from build123d import *

# Parameters (mm, degrees)
SKETCH1_W           = 55.5
SKETCH1_H           = 73.2
BOSS_EXTRUDE1_DEPTH = 4
SKETCH2_W           = 52.220028237
SKETCH2_H           = 5.163547568
BOSS_EXTRUDE2_DEPTH = 5
SKETCH3_W           = 43
SKETCH3_H           = 61
BOSS_EXTRUDE3_DEPTH = 3
SKETCH4_W           = 55.5
SKETCH4_H           = 73.2
BOSS_EXTRUDE4_DEPTH = 60


with BuildPart() as part:
    # Sketch1 → Boss-Extrude1 (new body)
    with BuildSketch(Plane.XY):
        Rectangle(SKETCH1_W, SKETCH1_H)
    extrude(amount=BOSS_EXTRUDE1_DEPTH)

    # Sketch2 → Boss-Extrude2 (add)
    with BuildSketch(Plane(origin=(0, 0, 0), x_dir=(-1, 0, 0), z_dir=(0, 0, -1))):
        with Locations((0.292276277, 32.734943074)):
            Rectangle(SKETCH2_W, SKETCH2_H)
    extrude(amount=BOSS_EXTRUDE2_DEPTH)

    # Sketch3 → Boss-Extrude3 (add)
    with BuildSketch(Plane.XY.offset(4)):
        Rectangle(SKETCH3_W, SKETCH3_H)
    extrude(amount=BOSS_EXTRUDE3_DEPTH)

    # Sketch4 → Boss-Extrude4 (add)
    with BuildSketch(Plane(origin=(0, 0, -5), x_dir=(-1, 0, 0), z_dir=(0, 0, -1))):
        Rectangle(SKETCH4_W, SKETCH4_H)
    extrude(amount=BOSS_EXTRUDE4_DEPTH)


solid = part.part
Work out the finished part from the listing and answer in its coordinate system (mm). A direction names the side the tool comes from. Give positions to 0.01 mm unless a question says otherwise; leave off trailing zeros. Order: outer loops, then holes, each group sorted by start corner. A loop starts at its lowest first (then second) coordinate and runs counter-clockwise, first axis right, second up. Notation, with made-up numbers: (-32, -29) - (-28, -29) arc R17 ccw to (-28, 2) - close; hole circle Ø3 at (33.25, 37). An arc over 180 degrees is marked (long way). Answer as CSV lines item,"result". Start each with the question number.
Q1. Find the intervals of material crossed by L1, parallel to Z at x = -7.5, y = 20; L2, parallel to Z at x = -25, y = -19; L3, parallel to Z at x = 14, y = 34.5, in increasing order. Write a range as [from, to].
Q2. The part is cut by section A-A (y = 14). Write down the section's boundary in (x, z), then the cut area to 3 significant figures.
Q3. The part is cut by section B-B (x = 24). Write down the section's boundary in (y, z), then the cut area to 3 significant figures.
Q4. Given pin 1 Ø5.5 at (y, z) = (33.5, -2) entering from -X; pin 2 Ø2.5 at (x, z) = (9.5, -2) entering from +Y; pin 3 Ø2.5 at (x, z) = (-8.5, 6) entering from -Y; pin 4 Ø3.5 at (y, z) = (2, 6) entering from -X, each flat-ended and moving along its own axis, determine where each tip first touches the part or whether it passes through.
Q5. The part is cut by section D-D (x = -5). Write down the section's boundary in (y, z), then the cut area to 3 significant figures.
Q6. For faces 1 (the face through (-21.5, 0, 5)), 2 (the face through (0, 35.317, -2)), 3 (the face through (0, 30.5, 5)), 4 (the face through (25.818, 33, -2)), 5 (the face through (21.5, 0, 5)), determine the directions among +Z, -Z, +X, -X, +Y, -Y from which every point of the face is accessible in a straight line to the end or side of a thin tool.
Q7. The mould has two halves that part along Z. Classify faces 6 (the face through (0, 1, -5)), 7 (the face through (0, 0, 7)), 8 (the face through (-27.75, -1, -35)): +Z half, -Z half, draft (parallel to the pull), parting line (faces both ways), or undercut.
Q8. The part is cut by section C-C (z = -3). Write down the section's boundary in (x, y), then the cut area to 3 significant figures.
Check result:
1,L1,"z = [-65, -5], [0, 7]"
1,L2,"z = [-65, -5], [0, 4]"
1,L3,"z = [-65, 4]"
2,outline,"(-27.75, -65) - (27.75, -65) - (27.75, -5) - (-27.75, -5) - close; (-27.75, 0) - (27.75, 0) - (27.75, 4) - (21.5, 4) - (21.5, 7) - (-21.5, 7) - (-21.5, 4) - (-27.75, 4) - close"
2,area,"3,680 mm²"
3,outline,"(-36.6, -65) - (36.6, -65) - (36.6, -5) - (35.32, -5) - (35.32, 0) - (36.6, 0) - (36.6, 4) - (-36.6, 4) - (-36.6, 0) - (30.15, 0) - (30.15, -5) - (-36.6, -5) - close"
3,area,"4,710 mm²"
4,pin 1,"stops at x = -27.75"
4,pin 2,"stops at y = 35.32"
4,pin 3,"stops at y = -30.5"
4,pin 4,"stops at x = -21.5"
5,outline,"(-36.6, -65) - (36.6, -65) - (36.6, -5) - (35.32, -5) - (35.32, 0) - (36.6, 0) - (36.6, 4) - (30.5, 4) - (30.5, 7) - (-30.5, 7) - (-30.5, 4) - (-36.6, 4) - (-36.6, 0) - (30.15, 0) - (30.15, -5) - (-36.6, -5) - close"
5,area,"4,890 mm²"
6,face 1,"+Z, -X, +Y, -Y"
6,face 2,"+X, -X, +Y"
6,face 3,"+Z, +X, -X, +Y"
6,face 4,"+X, +Y, -Y"
6,face 5,"+Z, +X, +Y, -Y"
7,face 6,"undercut"
7,face 7,"+Z half"
7,face 8,"draft"
8,outline,"(-26.4, 30.15) - (25.82, 30.15) - (25.82, 35.32) - (-26.4, 35.32) - close"
8,area,"270 mm²"
